Work out the finished part from the listing and answer in its coordinate system (mm). Face numbers are marked on the shaded views. A direction names the side the tool comes from. Give positions to 0.01 mm unless a question says otherwise; leave off trailing zeros. Loops run counter-clockwise (first coordinate to the right, second up) from the corner with the lowest first, then second, coordinate; pieces in that order, holes last. Notation, with made-up numbers: (-25, 25.5) - (20, 25.5) arc R21 cw to (20, 31.5) - close; hole circle Ø2 at (79.5, 34). An arc over 180 degrees is marked (long way). One line per question, with ' | ' between items.
from build123d import *

# Parameters (mm, degrees)
F0_W           = 56
F0_H           = 8
F1_DEPTH       = 20
F2_START       = -14.9
F2_DEPTH       = 4.8
F4_DEPTH       = 8
F5_R           = 2
F7_D           = 4.4
F7_CBORE_D     = 8.25
F7_CBORE_DEPTH = 4


# Not quite as in the source:
# - a feature of the source that left no trace in its solid (it failed there, or was rolled back) is left out


with BuildPart() as f1:
    # F0 (on Top) → F1 (new body, symmetric)
    with BuildSketch(Plane.XY):
        Polygon((-26.7077493668, 10), (-46.7077493668, 10), (-46.7077493668, -2), (13.2922506332, -2), (13.2922506332, 10), (-6.7077493668, 10), align=None)
        with Locations((-16.7077493668, 4)):
            Rectangle(F0_W, F0_H, mode=Mode.SUBTRACT)
    extrude(amount=F1_DEPTH, both=True)

    # F0 (on Top) → F2 (join)
    with BuildSketch(Plane.XY.offset(F2_START)):
        with Locations((-16.7077493668, 4)):
            Rectangle(F0_W, F0_H)
    extrude(amount=-F2_DEPTH)

    # F3 (on Front) → F4 (join)
    with BuildSketch(Plane.XZ):
        with BuildLine():
            Line((-26.7077493668, 57.6839694445), (-26.7077493668, -28.1024485154))
            ThreePointArc((-26.7077493668, -28.1024485154), (-16.7077493668, -38.1024485154), (-6.7077493668, -28.1024485154))
            Line((-6.7077493668, -28.1024485154), (-6.7077493668, 57.6839694445))
            ThreePointArc((-6.7077493668, 57.6839694445), (-16.7077493668, 67.6839694445), (-26.7077493668, 57.6839694445))
        make_face()
    extrude(amount=F4_DEPTH)

    # F5
    f5_edges = [f1.edges().sort_by_distance(p)[0] for p in [
        (-16.707749, 0, 67.683969),
        (-6.707749, 0, 38.841985),
        (-6.707749, 0, -24.051224),
        (-26.707749, 0, 38.841985),
        (-26.707749, 0, -24.051224),
    ]]
    fillet(f5_edges, radius=F5_R)

    # F7 (through all)
    with Locations(Plane(origin=(0, 0, 0), x_dir=(1, 0, 0), z_dir=(0, 1, 0))):
        with Locations((-16.7077493668, -57.6839694445), (-16.7077493668, 28.1024485154)):
            CounterBoreHole(F7_D / 2, F7_CBORE_D / 2, F7_CBORE_DEPTH)


solid = f1.part
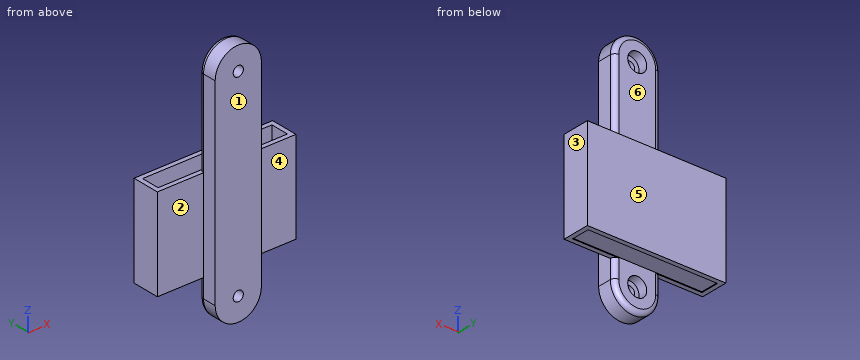
1. Find section A-A on z = -18.5. Write down the section's boundary in (x, y), then the cut area to 3 significant figures.
Evaluation:
outline: (-46.71, -2) - (-26.71, -2) - (-26.71, -8) - (-6.71, -8) - (-6.71, -2) - (13.29, -2) - (13.29, 10) - (-46.71, 10) - close | area: 840 mm2
2. Find section C-C on y = 1. Write down the section's boundary in (x, z), then the cut area to 3 significant figures.
Evaluation:
outline: (-46.71, -20) - (-44.71, -20) - (-44.71, -19.7) - (11.29, -19.7) - (11.29, -20) - (13.29, -20) - (13.29, 20) - (11.29, 20) - (11.29, -14.9) - (-44.71, -14.9) - (-44.71, 20) - (-46.71, 20) - close | area: 429 mm2
3. Flat-ended cylindrical pins translate along their axes: pin 1 (2.5 mm diameter, centred on x = -9, y = 4, fed in from -Z); pin 2 (2 mm diameter, centred on y = -3, z = -26, fed in from +X); pin 3 (4 mm diameter, centred on x = -15, z = 59, fed in from +Y). Find the tip coordinate at first contact, or state that the pin passes through.
Evaluation:
pin 1: z = -19.7 | pin 2: x = -6.71 | pin 3: y = 0
4. Find section D-D on x = 0.5. Write down the section's boundary in (y, z), then the cut area to 3 significant figures.
Evaluation:
outline: (-2, -20) - (0, -20) - (0, -19.7) - (8, -19.7) - (8, -20) - (10, -20) - (10, 20) - (8, 20) - (8, -14.9) - (0, -14.9) - (0, 20) - (-2, 20) - close | area: 198 mm2
5. Consider L1, parallel to X at y = 0.25, z = -8.5; L2, parallel to Y at x = -43.5, z = -1.5; L3, parallel to Y at x = -16.5, z = -13.5. Determine where each line is inside the solid, lowest interval first.
Evaluation:
L1: -46.71 to -44.71, 11.29 to 13.29 | L2: -2 to 0, 8 to 10 | L3: -8 to 0, 8 to 10
6. Which of the six approach directions +Z, -Z, +X, -X, +Y, -Y give full straight-line access (tool end or side, diameter ignored) to the marked faces 1 and 2?
Evaluation:
face 1: +Z, -Z, +X, -X, -Y | face 2: +Z, -Z, -X, -Y
7. Find section B-B on z = 8. Write down the section's boundary in (x, y).
Evaluation:
outline: (-46.71, -2) - (-26.71, -2) - (-26.71, -8) - (-6.71, -8) - (-6.71, -2) - (13.29, -2) - (13.29, 10) - (-46.71, 10) - close; hole (-44.71, 0) - (11.29, 0) - (11.29, 8) - (-44.71, 8) - close
8. Determine the mould class of the marked faces 3, 4, 5 and 6 for opening direction Y: +Y half, -Y half, draft (parallel to the pull), parting line (faces both ways), or undercut.
Evaluation:
face 3: draft | face 4: -Y half | face 5: +Y half | face 6: undercut
